Source: CAD feature listing. Evaluate the final solid. Frame: model axes, mm. Face numbers are marked on the shaded views. A direction names the side the tool comes from. Coordinates: 2 decimals unless noted, no trailing zeros. Order: outer loops, then holes, each group sorted by start corner. A loop starts at its lowest first (then second) coordinate and runs counter-clockwise, first axis right, second up.
```python
from build123d import *

# Parameters (mm, degrees)
F0_W      = 165
F0_H      = 45
F0_R      = 12.5
F1_DEPTH  = 1
F3_DEPTH  = 1
F4_DEPTH  = 25
F5_DEPTH  = 25
F6_R      = 13.5
F6_R_2    = 12.5
F7_DEPTH  = 5
F8_R      = 13.5
F8_R_2    = 5
F9_DEPTH  = 1
F11_DEPTH = 1
F12_W     = 1
F12_H     = 1
F12_H_2   = 36
F12_W_2   = 92
F13_DEPTH = 11
F14_W     = 94
F14_H     = 37
F15_DEPTH = 1
F16_W     = 1
F16_H     = 36
F17_DEPTH = 66
F18_W     = 26.2803444985
F18_H     = 1
F19_DEPTH = 3
F20_W     = 130
F20_H     = 1
F21_DEPTH = 78


with BuildPart() as f1:
    # F0 (on Front) → F1 (new body)
    with BuildSketch(Plane.XZ):
        Rectangle(F0_W, F0_H)
        with Locations((-65, 0)):
            Circle(F0_R, mode=Mode.SUBTRACT)
        with Locations((65, 0)):
            Circle(F0_R, mode=Mode.SUBTRACT)
    extrude(amount=F1_DEPTH)

    # F2 (on face) → F3 (join)
    with BuildSketch(Plane.XZ.offset(1)):
        with BuildLine():
            Line((68.3925151825, -19.0988145769), (65, -22.5))
            ThreePointArc((65, -22.5), (87.5, 0), (65, 22.5))
            Line((65, 22.5), (71.474224329, 16.2770561874))
            Line((71.474224329, 16.2770561874), (77.4062722921, 9.1145541519))
            Line((77.4062722921, 9.1145541519), (80.3926512599, 2.1407562308))
            Line((80.3926512599, 2.1407562308), (80.3926512599, -5.2317115478))
            Line((80.3926512599, -5.2317115478), (78.3914923668, -12.1520543471))
            Line((78.3914923668, -12.1520543471), (74.6632069349, -14.4081749022))
            Line((74.6632069349, -14.4081749022), (68.3925151825, -19.0988145769))
        make_face()
        with BuildLine():
            Line((-65, 14.9617949501), (-65, 22.5))
            ThreePointArc((-65, 22.5), (-87.5, 0), (-65, -22.5))
            Line((-65, -22.5), (-67.4760043621, -15.6979020685))
            Line((-67.4760043621, -15.6979020685), (-72.8440880775, -12.9142012447))
            Line((-72.8440880775, -12.9142012447), (-76.5851810575, -7.8018400818))
            Line((-76.5851810575, -7.8018400818), (-79.5639529824, 0))
            Line((-79.5639529824, 0), (-79.5639529824, 6.4657721668))
            Line((-79.5639529824, 6.4657721668), (-75.4495188594, 11.7608513683))
            Line((-75.4495188594, 11.7608513683), (-65, 14.9617949501))
        make_face()
    extrude(amount=-F3_DEPTH)

    # F2 (on face) → F4 (cut)
    with BuildSketch(Plane.XZ.offset(1)):
        with BuildLine():
            Line((-82.5, 22.5), (-82.5, 14.1421356237))
            ThreePointArc((-82.5, 14.1421356237), (-74.6966991411, 20.3033008589), (-65, 22.5))
            Line((-65, 22.5), (-82.5, 22.5))
        make_face()
    extrude(amount=-F4_DEPTH, mode=Mode.SUBTRACT)

    # F2 (on face) → F5 (cut)
    with BuildSketch(Plane.XZ.offset(1)):
        with BuildLine():
            ThreePointArc((82.5, -14.1421356237), (74.6966991411, -20.3033008589), (65, -22.5))
            Line((65, -22.5), (82.5, -22.5))
            Line((82.5, -22.5), (82.5, -14.1421356237))
        make_face()
        with BuildLine():
            ThreePointArc((65, 22.5), (74.6966991411, 20.3033008589), (82.5, 14.1421356237))
            Line((82.5, 14.1421356237), (82.5, 22.5))
            Line((82.5, 22.5), (65, 22.5))
        make_face()
        with BuildLine():
            Line((-82.5, -22.5), (-65, -22.5))
            ThreePointArc((-65, -22.5), (-74.6966991411, -20.3033008589), (-82.5, -14.1421356237))
            Line((-82.5, -14.1421356237), (-82.5, -22.5))
        make_face()
    extrude(amount=-F5_DEPTH, mode=Mode.SUBTRACT)

    # F6 (on face) → F7 (join)
    with BuildSketch(Plane.XZ.offset(1)):
        with Locations((-65, 0)):
            Circle(F6_R)
        with Locations((-65, 0)):
            Circle(F6_R_2, mode=Mode.SUBTRACT)
        with Locations((65, 0)):
            Circle(F6_R)
        with Locations((65, 0)):
            Circle(F6_R_2, mode=Mode.SUBTRACT)
    extrude(amount=F7_DEPTH)

    # F8 (on face) → F9 (join)
    with BuildSketch(Plane.XZ.offset(6)):
        with Locations((-65, 0)):
            Circle(F8_R)
        with Locations((-65, 0)):
            Circle(F8_R_2, mode=Mode.SUBTRACT)
        with Locations((65, 0)):
            Circle(F8_R)
        with Locations((65, 0)):
            Circle(F8_R_2, mode=Mode.SUBTRACT)
    extrude(amount=F9_DEPTH)

    # F10 (on face) → F11 (join)
    with BuildSketch(Plane.XZ.offset(1)):
        Polygon((-81.9395110011, 0), (-87.5, 0), (-87.5, -22.5), (-65, -22.5), (-65, -18.5897927731), (-73.3228996396, -16.0001199692), (-80.1934376359, -9.6208481118), align=None)
    extrude(amount=-F11_DEPTH)

    # F12 (on face) → F13 (join)
    with BuildSketch(Plane.XZ.offset(1)):
        with Locations((46.5, -14)):
            Rectangle(F12_W, F12_H)
        with Locations((46.5, 4.5)):
            Rectangle(F12_W, F12_H_2)
        with Locations((0, -14)):
            Rectangle(F12_W_2, F12_H)
        with Locations((-46.5, -14)):
            Rectangle(F12_W, F12_H)
        with Locations((-46.5, 4.5)):
            Rectangle(F12_W, F12_H_2)
    extrude(amount=F13_DEPTH)

    # F14 (on face) → F15 (join)
    with BuildSketch(Plane.XZ.offset(12)):
        with Locations((0, 4)):
            Rectangle(F14_W, F14_H)
    extrude(amount=F15_DEPTH)

    # F16 (on face) → F17 (join)
    with BuildSketch(Plane.XZ.offset(13)):
        with Locations((-46.5, 4.5)):
            Rectangle(F16_W, F16_H)
        with Locations((46.5, 4.5)):
            Rectangle(F16_W, F16_H)
    extrude(amount=F17_DEPTH)

    # F18 (on face) → F19 (join)
    with BuildSketch(Plane.XZ.offset(1)):
        with Locations((0.058112666, -11)):
            Rectangle(F18_W, F18_H)
    extrude(amount=F19_DEPTH)

    # F20 (on face) → F21 (join)
    with BuildSketch(Plane.XZ.offset(1)):
        with Locations((0, 22)):
            Rectangle(F20_W, F20_H)
        with BuildLine():
            ThreePointArc((65, -22.5), (87.5, 0), (65, 22.5))
            Line((65, 22.5), (65, 21.5))
            ThreePointArc((65, 21.5), (80.2027957955, 15.2027957955), (86.5, 0))
            ThreePointArc((86.5, 0), (80.2027957955, -15.2027957955), (65, -21.5))
            Line((65, -21.5), (65, -22.5))
        make_face()
        with BuildLine():
            Line((65, 21.5), (-65, 21.5))
            ThreePointArc((-65, 21.5), (-80.2027957955, 15.2027957955), (-86.5, 0))
            Line((-86.5, 0), (-86.5, -21.5))
            Line((-86.5, -21.5), (62.4147094786, -21.5))
            Line((62.4147094786, -21.5), (65, -21.5))
            ThreePointArc((65, -21.5), (43.5, 0), (65, 21.5))
        make_face()
        Polygon((-86.5, -22.5), (65, -22.5), (65, -21.5), (62.4147094786, -21.5), (-86.5, -21.5), align=None)
        Polygon((-86.5, -21.5), (-86.5, 0), (-87.5, 0), (-87.5, -22.5), (-86.5, -22.5), align=None)
    extrude(amount=F21_DEPTH)


solid = f1.part
```
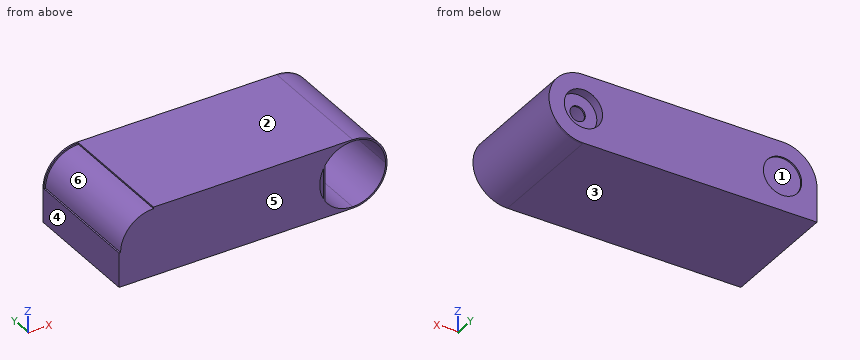
Q1. Section query A-A on y = -47. Output: boundary loops of the cut face in (x, z).
Solutions:
outline: (-87.5, -22.5) - (65, -22.5) arc R22.5 ccw to (65, 22.5) - (-65, 22.5) - (-65, 21.5) arc R21.5 ccw to (-86.5, 0) - (-87.5, 0) - close; hole (46, -10.06) - (46, 10.06) arc R21.5 ccw to start; hole (47, -11.76) arc R21.5 ccw (long way) to (47, 11.76) - close
Q2. Material intervals for line 1 along Z through (x, y) = (65, -6.5); line 2 along Z through (x, y) = (65, -1.6); line 3 along X through (y, z) = (-21.5, 3), sorted ascending.
Solutions:
line 1: z = -22.5 to -21.5, -13.5 to -5, 5 to 13.5, 21.5 to 22.5
line 2: z = -22.5 to -21.5, -13.5 to -12.5, 12.5 to 13.5, 21.5 to 22.5
line 3: x = -86.29 to 43.71, 46 to 47, 86.29 to 87.3
Q3. Pull-direction query (Z, two-part tool) for the marked faces 1, 2, 3 and 4; classes: pulls with the +Z half, pulls with the -Z half, needs draft (parallel to the pull), parting line crosses it, or undercut.
Solutions:
face 1: undercut
face 2: pulls with the +Z half
face 3: pulls with the -Z half
face 4: needs draft
Q4. Pin query (flat end, axial travel): P1, Ø12.5, axis at x = 65.5, z = 2, coming from the +Y side; P2, Ø8, axis at x = 65, z = 0, coming from the +Y side; P3, Ø1, axis at y = -52.5, z = 10, coming from the +X side; P4, Ø5.5, axis at y = -7.5, z = 1, coming from the -X side. Return the tip coordinate at first contact, or that it passes through.
Solutions:
P1: stops at y = -6
P2: passes through
P3: stops at x = 85.4
P4: stops at x = -87.5
Q5. Set-up query: the marked faces 5 and 6. Return all of +Z, -Z, +X, -X, +Y, -Y with unobstructed straight access to the full face (end or side cutting, diameter ignored); none if empty.
Solutions:
face 5: +Z, -Z, +X, -X, -Y
face 6: +Z, -X, -Y
Q6. Section query B-B on x = 74. Output: boundary loops of the cut face in (y, z), plus the area to 3 significant figures.
Solutions:
outline: (-79, -20.62) - (0, -20.62) - (0, -8.67) - (-6, -8.67) - (-6, 8.67) - (0, 8.67) - (0, 20.62) - (-79, 20.62) - (-79, 19.53) - (-1, 19.53) - (-1, 10.06) - (-7, 10.06) - (-7, -10.06) - (-1, -10.06) - (-1, -19.53) - (-79, -19.53) - close
area: 229 mm2
